from build123d import *

# Parameters (mm, degrees)
RESSALTO_EXTRUS_O1_DEPTH = 175
CORTE_EXTRUS_O1_DEPTH    = 50
CORTE_EXTRUS_O2_DEPTH    = 1.5


with BuildPart() as part:
    # Esboço1 → Ressalto-extrusão1 (new, symmetric)
    with BuildSketch(Plane(origin=(0, 0, 0), x_dir=(0, 0, -1), z_dir=(1, 0, 0))):
        Polygon((0, 20), (0, -20), (-20, -20), (-20, -18.5), (-1.5, -18.5), (-1.5, 18.5), (-20, 18.5), (-20, 20), align=None)
    extrude(amount=RESSALTO_EXTRUS_O1_DEPTH, both=True)

    # Esboço2 → Corte-extrusão1 (cut, symmetric)
    with BuildSketch(Plane(origin=(0, 20, 0), x_dir=(1, 0, 0), z_dir=(0, 1, 0))):
        Polygon((-175, 0), (-155, -20), (-175, -20), align=None)
        Polygon((175, 0), (155, -20), (175, -20), align=None)
    extrude(amount=CORTE_EXTRUS_O1_DEPTH, both=True, mode=Mode.SUBTRACT)

    # Esboço3 → Corte-extrusão2 (cut)
    with BuildSketch(Plane.XZ.offset(20)):
        with BuildLine():
            Line((-103.5, 11), (-103.5, 8))
            ThreePointArc((-103.5, 8), (-100, 4.5), (-96.5, 8))
            Line((-96.5, 8), (-96.5, 11))
            ThreePointArc((-96.5, 11), (-100, 14.5), (-103.5, 11))
        make_face()
        with BuildLine():
            Line((96.5, 8), (96.5, 11))
            ThreePointArc((96.5, 11), (100, 14.5), (103.5, 11))
            Line((103.5, 11), (103.5, 8))
            ThreePointArc((103.5, 8), (100, 4.5), (96.5, 8))
        make_face()
    extrude(amount=-CORTE_EXTRUS_O2_DEPTH, mode=Mode.SUBTRACT)


solid = part.part
Build history of the part. All positions in model axes, mm. A direction names the side the tool comes from. Give positions to 0.01 mm unless a question says otherwise; leave off trailing zeros. Order: outer loops, then holes, each group sorted by start corner. A loop starts at its lowest first (then second) coordinate and runs counter-clockwise, first axis right, second up. Notation, with made-up numbers: M -25,75 L -1,75 A21 ccw -1,93 Z; hole C -9,30 d4. An arc over 180 degrees is marked long. Use one line per item in the form item = value.
Q1. Wall check: probe 1 along Y at (x, z) = (-141, 4.25); probe 2 along Z at (x, y) = (-67, 16.5); probe 3 along X at (y, z) = (-0.5, 1). Give the ranges that are in metal, low to high.
Conclusion:
probe_1 = -20 to -18.5, 18.5 to 20
probe_2 = 0 to 1.5
probe_3 = -174 to 174
Q2. Pin check, flat tips, straight feed: P1, Ø10, axis at x = -4.5, y = -15.5, coming from the -Z side; P2, Ø18.5, axis at x = 7, y = 1.5, coming from the +Z side; P3, Ø1.2, axis at y = -19.5, z = 10, coming from the +X side; P4, Ø0.8, axis at y = -19.5, z = 10, coming from the -X side. Stop position of each tip, or through.
Conclusion:
P1 = 0
P2 = 1.5
P3 = 165.6
P4 = -165.4
Q3. Pull direction Y, two halves, no side cores. Call faces 3 (the flat face through (2, 0, 0)), 4 (the flat face through (2, 20, 10)), 5 (the flat face through (2, 0, 1.5)): released by +Y, released by -Y, zero draft, split by the parting line, or undercut.
Conclusion:
face_3 = zero draft
face_4 = released by +Y
face_5 = undercut
Q4. Which spindle directions (+Z, -Z, +X, -X, +Y, -Y) get a long thin tool onto all of the face, cutting with end or side? Do faces 1 (the flat face through (174, 0, 1)), 2 (the flat face through (2, -18.5, 11)). Say none if no direction does.
Conclusion:
face_1 = +Z, +X, +Y, -Y
face_2 = +Z, +X, -X
Q5. Slice it at B-B, the plane x = -34.5. Write the cut outline in (y, z), and give its area (4 significant figures).
Conclusion:
outline = M -20,0 L 20,0 L 20,20 L 18.5,20 L 18.5,1.5 L -18.5,1.5 L -18.5,20 L -20,20 Z
area = 115.5 mm2
Q6. Slice it at A-A, the plane x = -100. Write the cut outline in (y, z), and give its area (4 significant figures).
Conclusion:
outline = M -20,0 L 20,0 L 20,20 L 18.5,20 L 18.5,1.5 L -18.5,1.5 L -18.5,4.5 L -20,4.5 Z; M -20,14.5 L -18.5,14.5 L -18.5,20 L -20,20 Z
area = 100.5 mm2
Q7. Slice it at C-C, the plane y = 15.5. Write the cut outline in (x, z).
Conclusion:
outline = M -175,0 L 175,0 L 173.5,1.5 L -173.5,1.5 Z
